from build123d import *

# Parameters (mm, degrees)
F0_W     = 100
F0_H     = 120
F1_DEPTH = 100
F2_T     = -3
F3_W     = 100
F3_H     = 60
F4_DEPTH = 3
F5_R     = 6
F6_DEPTH = 25


with BuildPart() as f1:
    # F0 (on Top) → F1 (new body)
    with BuildSketch(Plane.XY):
        Rectangle(F0_W, F0_H)
    extrude(amount=F1_DEPTH)

    # F2
    f2_openings = [f1.faces().sort_by_distance(p)[0] for p in [
        (0, 0, 100),
    ]]
    offset(amount=F2_T, openings=f2_openings)

    # F3 (on face) → F4 (join)
    with BuildSketch(Plane.XY.offset(100)):
        with Locations((0, 30)):
            Rectangle(F3_W, F3_H)
    extrude(amount=-F4_DEPTH)

    # F5 (on face) → F6 (cut)
    with BuildSketch(Plane.XY.offset(100)):
        with Locations((0, 30)):
            Circle(F5_R)
        with Locations((35, 30)):
            Circle(F5_R)
        with Locations((-35, 30)):
            Circle(F5_R)
        with Locations((-35, 50)):
            Circle(F5_R)
        with Locations((0, 50)):
            Circle(F5_R)
        with Locations((35, 50)):
            Circle(F5_R)
        with Locations((-35, 10)):
            Circle(F5_R)
        with Locations((0, 10)):
            Circle(F5_R)
        with Locations((35, 10)):
            Circle(F5_R)
    extrude(amount=-F6_DEPTH, mode=Mode.SUBTRACT)


solid = f1.part
Build history of the part. All positions in model axes, mm. A direction names the side the tool comes from. Round coordinates to 2 decimals unless told otherwise and drop trailing zeros. Loops run counter-clockwise (first coordinate to the right, second up) from the corner with the lowest first, then second, coordinate; pieces in that order, holes last. Notation, with made-up numbers: (73, -25.75) -> (111, -25.75) arc R33 ccw to (111, 12.25) -> close; hole circle Ø10 at (73, -27). An arc over 180 degrees is marked (long way). Use CSV: the item, a comma, the result in double quotes. Start each with the question number.
Q1. Which spindle directions (+Z, -Z, +X, -X, +Y, -Y) get a long thin tool onto all of the face, cutting with end or side? Do faces 1 (the face through (-1, 57, 49)), 2 (the face through (33.699, 24.143, 98.521)), 3 (the face through (-1, 60, 49)). Say none if no direction does.
Q2. Drill centre lines: L1, parallel to Y at x = -35, z = 99.15; L2, parallel to Y at x = -20, z = 77.5; L3, parallel to X at y = 39.5, z = 16.5. Where is each one in solid material? Low to high.
Q3. Flat gauge pin, fed straight in: pin 1 Ø9.5 at (x, y) = (-35, 10) entering from +Z. Where does the tip first touch, or does it go through?
Q4. Saw through at D-D on y = 50. Give the cut face in (x, z), and give its area (3 significant figures).
Q5. Saw through at A-A on z = 63.5. Give the cut face in (x, y).
Q6. Saw through at B-B on y = 37.5. Give the cut face in (x, z).
Q7. Saw through at C-C on x = 0. Give the cut face in (y, z).
Q8. Mould opens along Z. For faces 4 (the face through (-1, 23, 97)), 5 (the face through (-12, 28, 100)), 6 (the face through (-50, -1, 49)) say: +Z half, -Z half, draft (parallel to the pull), parting line (faces both ways), or undercut.
Solutions:
1,face 1,"none"
1,face 2,"+Z"
1,face 3,"+Z, -Z, +X, -X, +Y"
2,L1,"y = -60 to -57, 0 to 4, 16 to 24, 36 to 44, 56 to 60"
2,L2,"y = -60 to -57, 57 to 60"
2,L3,"x = -50 to -47, 47 to 50"
3,pin 1,"stops at z = 3"
4,outline,"(-50, 0) -> (50, 0) -> (50, 100) -> (41, 100) -> (41, 97) -> (47, 97) -> (47, 3) -> (-47, 3) -> (-47, 97) -> (-41, 97) -> (-41, 100) -> (-50, 100) -> close; (-29, 97) -> (-6, 97) -> (-6, 100) -> (-29, 100) -> close; (6, 97) -> (29, 97) -> (29, 100) -> (6, 100) -> close"
4,area,"1,060 mm^2"
5,outline,"(-50, -60) -> (50, -60) -> (50, 60) -> (-50, 60) -> close; hole (-47, -57) -> (47, -57) -> (47, 57) -> (-47, 57) -> close"
6,outline,"(-50, 0) -> (50, 0) -> (50, 100) -> (-50, 100) -> close; hole (-47, 3) -> (47, 3) -> (47, 97) -> (-47, 97) -> close"
7,outline,"(-60, 0) -> (60, 0) -> (60, 100) -> (56, 100) -> (56, 97) -> (57, 97) -> (57, 3) -> (-57, 3) -> (-57, 100) -> (-60, 100) -> close; (0, 97) -> (4, 97) -> (4, 100) -> (0, 100) -> close; (16, 97) -> (24, 97) -> (24, 100) -> (16, 100) -> close; (36, 97) -> (44, 97) -> (44, 100) -> (36, 100) -> close"
8,face 4,"undercut"
8,face 5,"+Z half"
8,face 6,"draft"
